The model under review builds one solid part; all positions refer to its coordinate system, in mm. Face numbers are marked on the shaded views. Round coordinates to 2 decimals unless told otherwise and drop trailing zeros. Write each loop counter-clockwise with the first axis right and the second up, starting at its lowest first coordinate (ties: lowest second). Pieces come first, ordered by that corner, then holes. Notation, with made-up numbers: (-35.75, 12) -> (-8.75, 12) arc R34 cw to (-8.75, 43) -> close; hole circle Ø3 at (-15, 38.5). An arc over 180 degrees is marked (long way). Answer in a Markdown table with one row per item. Add a question column.
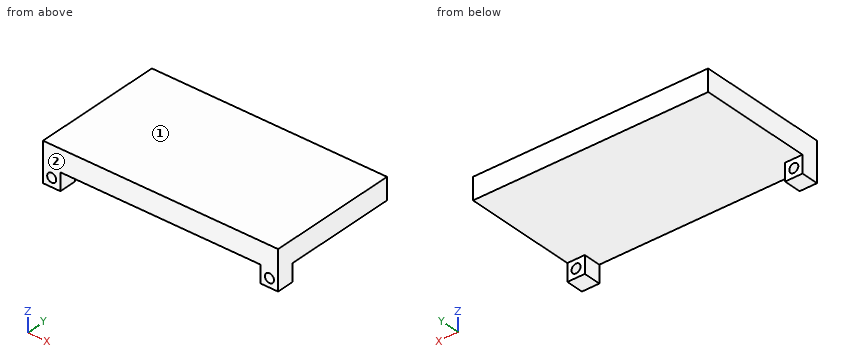
```python
from build123d import *

# Parameters (mm, degrees)
F0_W     = 137.16
F0_H     = 12.7
F1_DEPTH = 76.2
F2_W     = 10.16
F2_H     = 10.16
F3_DEPTH = 10.16
F4_R     = 2.6416
F5_DEPTH = 25.4


with BuildPart() as f1:
    # F0 (on Front) → F1 (new body)
    with BuildSketch(Plane.XZ):
        with Locations((0.306241, 0)):
            Rectangle(F0_W, F0_H)
    extrude(amount=F1_DEPTH)

    # F2 (on face) → F3 (join)
    with BuildSketch(Plane.XZ.offset(76.2)):
        with Locations((-63.193759, -11.43)):
            Rectangle(F2_W, F2_H)
        with Locations((63.806241, -11.43)):
            Rectangle(F2_W, F2_H)
    extrude(amount=-F3_DEPTH)

    # F4 (on face) → F5 (cut)
    with BuildSketch(Plane.XZ.offset(76.2)):
        with Locations((-63.193759, -11.43)):
            Circle(F4_R)
        with Locations((63.806241, -11.43)):
            Circle(F4_R)
    extrude(amount=-F5_DEPTH, mode=Mode.SUBTRACT)


solid = f1.part
```
1. Mouldability with a two-part tool opening along Z and no side actions: class the marked faces 1 and 2 as pulls with the +Z half, pulls with the -Z half, needs draft (parallel to the pull), parting line crosses it, or undercut.
2. Insertion check: pin 1 Ø8 at (x, z) = (-63, -14) entering from +Y; pin 2 Ø8 at (x, y) = (13.5, -65.5) entering from -Z. Each pin has a flat end and moves straight along its axis. Give the tip position at first contact, or say it passes through.
3. Add section B-B on x = 13. Write out the cut boundary in (y, z), plus the area to 3 significant figures.
4. For L1, parallel to Z at x = 7, y = -16.5, list the stretches that pass through material, from the lowest coordinate up.
5. Add section C-C on y = -47. Write out the cut boundary in (x, z).
6. Add section A-A on z = -11.43. Write out the cut boundary in (x, y).
Filled in:
| question | item | result |
|---|---|---|
| 1 | face 1 | pulls with the +Z half |
| 1 | face 2 | needs draft |
| 2 | pin 1 | y = -66.04 |
| 2 | pin 2 | z = -6.35 |
| 3 | outline | (-76.2, -6.35) -> (0, -6.35) -> (0, 6.35) -> (-76.2, 6.35) -> close |
| 3 | area | 968 mm² |
| 4 | L1 | -6.35 to 6.35 |
| 5 | outline | (-68.27, -6.35) -> (68.89, -6.35) -> (68.89, 6.35) -> (-68.27, 6.35) -> close |
| 6 | outline | (-68.27, -76.2) -> (-65.84, -76.2) -> (-65.84, -66.04) -> (-68.27, -66.04) -> close; (-60.55, -76.2) -> (-58.11, -76.2) -> (-58.11, -66.04) -> (-60.55, -66.04) -> close; (58.73, -76.2) -> (61.16, -76.2) -> (61.16, -66.04) -> (58.73, -66.04) -> close; (66.45, -76.2) -> (68.89, -76.2) -> (68.89, -66.04) -> (66.45, -66.04) -> close |
